```python
from build123d import *

# Parameters (mm, degrees)
F0_R     = 2.921
F1_DEPTH = 5.842
F3_DEPTH = 5.842


with BuildPart() as f1:
    # F0 (on Top) → F1 (new body)
    with BuildSketch(Plane.XY):
        with BuildLine():
            Line((0, 25.4), (0, 0))
            Line((0, 0), (25.4, 0))
            ThreePointArc((25.4, 0), (17.9605122421, 17.9605122421), (0, 25.4))
        make_face()
        with Locations((8.9802561211, 8.9802561211)):
            Circle(F0_R, mode=Mode.SUBTRACT)
    extrude(amount=F1_DEPTH)

    # F2 (on face) → F3 (cut, through all)
    with BuildSketch(Plane.XY.offset(5.842)):
        with BuildLine():
            Line((0, 0), (3.6948170712, 0))
            ThreePointArc((3.6948170712, 0), (2.2450640303, 2.2450640303), (0, 3.6948170712))
            Line((0, 3.6948170712), (0, 0))
        make_face()
    extrude(amount=-F3_DEPTH, mode=Mode.SUBTRACT)


solid = f1.part
```
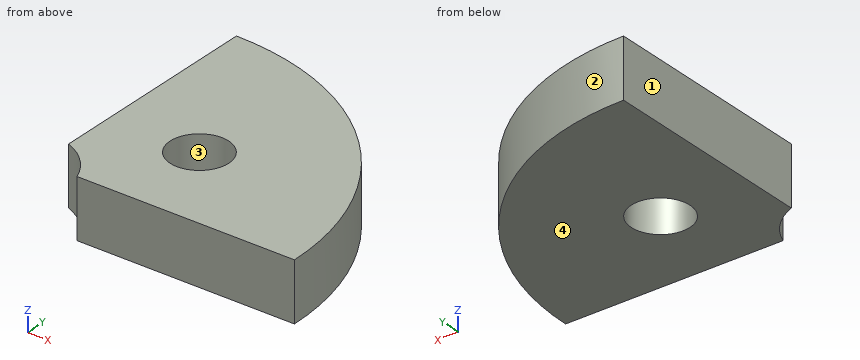
Verification items for the finished model (mm, model axes). Face numbers are marked on the shaded views. Give positions to 0.01 mm unless a question says otherwise; leave off trailing zeros. Order: outer loops, then holes, each group sorted by start corner. A loop starts at its lowest first (then second) coordinate and runs counter-clockwise, first axis right, second up. Notation, with made-up numbers: (-18.75, -15.75) - (7.25, -15.75) arc R26 cw to (7.25, 21.25) - close; hole circle Ø2 at (20.5, 49.5). An arc over 180 degrees is marked (long way). Answer as CSV lines item,"result". Start each with the question number.
Item 1: Section check C-C, the plane z = 0.7. Record the boundary of the cut face in (x, y), plus the area to 3 significant figures.
Item 2: Mould release check, pull along X, two halves, no side actions. Record for the marked faces 1, 2, 3 and 4: released by +X, released by -X, zero draft, split by the parting line, or undercut.
Item 3: Section check B-B, the plane x = 7.5. Record the boundary of the cut face in (y, z), plus the area to 3 significant figures.
Item 4: Section check D-D, the plane y = 22. Record the boundary of the cut face in (x, z).
Item 5: Section check A-A, the plane y = 10.75. Record the boundary of the cut face in (x, z).
Item 6: Gauge pin test, flat ends, axial feed: pin 1 (1.5 mm diameter, centred on y = 18, z = 1, fed in from +X); pin 2 (1 mm diameter, centred on x = 14.5, z = 0.5, fed in from +Y). Record the tip position at first contact, or that the pin passes through.
Item 7: Material ranges on L1, parallel to Y at x = 11, z = 1.95; L2, parallel to Y at x = 7.25, z = 4.5; L3, parallel to X at y = 9.25, z = 0.55, recorded low to high.
Filled in:
1,outline,"(0, 3.69) arc R6.35 cw to (3.69, 0) - (25.4, 0) arc R25.4 ccw to (0, 25.4) - close; hole circle Ø5.84 at (8.98, 8.98)"
1,area,"471 mm^2"
2,face 1,"released by -X"
2,face 2,"released by +X"
2,face 3,"undercut"
2,face 4,"zero draft"
3,outline,"(0, 0) - (6.46, 0) - (6.46, 5.84) - (0, 5.84) - close; (11.5, 0) - (24.27, 0) - (24.27, 5.84) - (11.5, 5.84) - close"
3,area,"112 mm^2"
4,outline,"(0, 0) - (12.69, 0) - (12.69, 5.84) - (0, 5.84) - close"
5,outline,"(0, 0) - (6.66, 0) - (6.66, 5.84) - (0, 5.84) - close; (11.3, 0) - (23.01, 0) - (23.01, 5.84) - (11.3, 5.84) - close"
6,pin 1,"x = 18.64"
6,pin 2,"y = 21.19"
7,L1,"0 to 6.87, 11.09 to 22.89"
7,L2,"0 to 6.63, 11.33 to 24.34"
7,L3,"0 to 6.07, 11.89 to 23.66"
